For this review, take the finished solid that the model builds, in its own axes (mm). Face numbers are marked on the shaded views. Coordinates: 2 decimals unless noted, no trailing zeros.
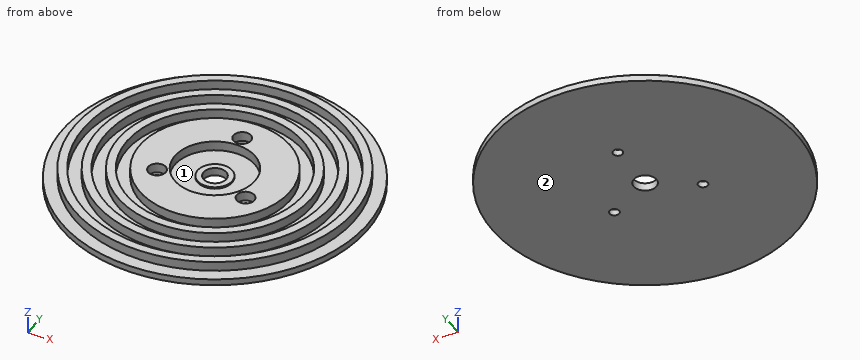
from build123d import *

# Parameters (mm, degrees)
F2_R     = 1.5
F3_DEPTH = 5.001
F4_R     = 2.75
F5_DEPTH = 3


with BuildPart() as f1:
    # F0 (on Front) → F1 (revolve)
    with BuildSketch(Plane.XZ):
        Polygon((3.55, 2.5), (3.55, 0), (47.5, 0), (47.5, 2), (43.5, 2), (43.5, 5), (40.8, 5), (40.8, 2), (36.8, 2), (36.8, 5), (34.1, 5), (34.1, 2), (30.1, 2), (30.1, 5), (27.4, 5), (27.4, 2), (23.4, 2), (23.4, 5), (12.5, 5), (12.5, 2), (5.4, 2), (5.4, 2.5), align=None)
    revolve(axis=Axis((0, 0, 0.333373), (0, 0, -1)))

    # F2 (on Top) → F3 (cut, through all)
    with BuildSketch(Plane.XY):
        with Locations((0, 16)):
            Circle(F2_R)
        with Locations((-13.856406, -8)):
            Circle(F2_R)
        with Locations((13.856406, -8)):
            Circle(F2_R)
    extrude(amount=F3_DEPTH, mode=Mode.SUBTRACT)

    # F4 (on face) → F5 (cut)
    with BuildSketch(Plane.XY.offset(5)):
        with Locations((0, 16)):
            Circle(F4_R)
        with Locations((-13.856406, -8)):
            Circle(F4_R)
        with Locations((13.856406, -8)):
            Circle(F4_R)
    extrude(amount=-F5_DEPTH, mode=Mode.SUBTRACT)


solid = f1.part
1. To check wall thickness, follow L1, parallel to Y at x = 0, z = 1.1; L2, parallel to X at y = 0, z = 1.55; L3, parallel to X at y = -8, z = 1.35. State the ranges of each line that lie inside material, in increasing order.
Answer below:
L1: y = -47.5 to -3.55, 3.55 to 14.5, 17.5 to 47.5
L2: x = -47.5 to -3.55, 3.55 to 47.5
L3: x = -46.82 to -15.36, -12.36 to 12.36, 15.36 to 46.82
2. Take a section at A-A, the plane z = 3.4. Give the number of separate pieces and of enclosed holes in the cut face, plus the area to 3 significant figures.
Answer below:
separate pieces: 4
enclosed holes: 7
area: 2,960 mm2
3. The part is to be moulded in two halves that separate along Y. For the marked faces 1 and 2, say which applies: +Y half, -Y half, draft (parallel to the pull), parting line (faces both ways), or undercut.
Answer below:
face 1: undercut
face 2: draft
4. Clearance check with flat-ended pins moving along their axes: pin 1 Ø1.6 at (x, y) = (1, 16.5) entering from +Z; pin 2 Ø1 at (y, z) = (28, 1) entering from +X; pin 3 Ø3 at (x, z) = (-10.5, 1.5) entering from +Y. State where each tip first meets the part, or that it passes through.
Answer below:
pin 1: stops at z = 2
pin 2: stops at x = 38.73
pin 3: stops at y = 46.64
